Check sheet for the modelled part. Datum: model origin and axes. Units: mm. Face numbers are marked on the shaded views. A direction names the side the tool comes from. Coordinates: 2 decimals unless noted, no trailing zeros. Write each loop counter-clockwise with the first axis right and the second up, starting at its lowest first coordinate (ties: lowest second). Pieces come first, ordered by that corner, then holes. Notation, with made-up numbers: (29.5, -22.75) - (85.5, -22.75) arc R13 ccw to (85.5, -7.75) - close; hole circle Ø3 at (-1, 43). An arc over 180 degrees is marked (long way). Answer as CSV lines item,"result". Start each with the question number.
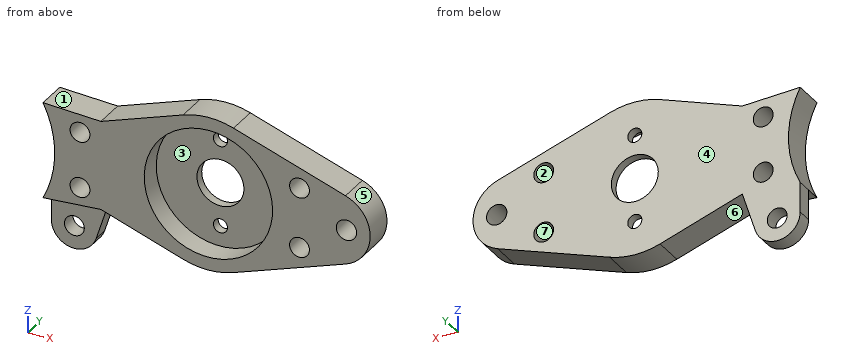
from build123d import *

# Parameters (mm, degrees)
SKETCH1_R           = 1.9
SKETCH1_R_2         = 1.95
BOSS_EXTRUDE1_DEPTH = 6
SKETCH2_R           = 12.3
CUT_EXTRUDE1_DEPTH  = 4.3
SKETCH5_R           = 1.35
SKETCH5_R_2         = 4.5
CUT_EXTRUDE3_DEPTH  = 6
SKETCH6_R           = 1.9
BOSS_EXTRUDE3_DEPTH = 3


with BuildPart() as part:
    # Sketch1 → Boss-Extrude1 (new body)
    with BuildSketch(Plane(origin=(0, 0, 0), x_dir=(1, 0, 0), z_dir=(0, 1, 0))):
        with BuildLine():
            Line((11.089751242, 8.53), (0, 9.208278243))
            ThreePointArc((0, 9.208278243), (2.245912814, 0), (0, -9.208278243))
            Line((0, -9.208278243), (11.089751242, -8.53))
            Line((11.089751242, -8.53), (26.847851363, -13.985564185))
            ThreePointArc((26.847851363, -13.985564185), (31.672879121, -14.799990383), (36.499751242, -13.996567436))
            Line((36.499751242, -13.996567436), (57.964751242, -6.619998112))
            ThreePointArc((57.964751242, -6.619998112), (62.689751242, 0), (57.964751242, 6.619998112))
            Line((57.964751242, 6.619998112), (36.499751242, 13.996567436))
            ThreePointArc((36.499751242, 13.996567436), (31.672879121, 14.799990383), (26.847851363, 13.985564185))
            Line((26.847851363, 13.985564185), (11.089751242, 8.53))
        make_face()
        with Locations(Location((7.089751242, -5.35, 0), (0, 0, 270))):
            Circle(SKETCH1_R, mode=Mode.SUBTRACT)
        with Locations(Location((7.089751242, 5.35, 0), (0, 0, 270))):
            Circle(SKETCH1_R, mode=Mode.SUBTRACT)
        with Locations(Location((49.14768086, 5.75, 0), (0, 0, 270))):
            Circle(SKETCH1_R, mode=Mode.SUBTRACT)
        with Locations(Location((49.14768086, -5.75, 0), (0, 0, 270))):
            Circle(SKETCH1_R, mode=Mode.SUBTRACT)
        with Locations(Location((58.14768086, 0, 0), (0, 0, 270))):
            Circle(SKETCH1_R_2, mode=Mode.SUBTRACT)
    extrude(amount=BOSS_EXTRUDE1_DEPTH)

    # Sketch2 → Cut-Extrude1 (cut)
    with BuildSketch(Plane(origin=(0, 0, 0), x_dir=(1, 0, 0), z_dir=(0, 1, 0))):
        with Locations(Location((31.689751242, 0, 0), (0, 0, 270))):
            Circle(SKETCH2_R)
    extrude(amount=CUT_EXTRUDE1_DEPTH, mode=Mode.SUBTRACT)

    # Sketch5 → Cut-Extrude3 (cut)
    with BuildSketch(Plane(origin=(0, 0, 0), x_dir=(1, 0, 0), z_dir=(0, 1, 0))):
        with Locations(Location((31.689751242, 8.35, 0), (0, 0, 270))):
            Circle(SKETCH5_R)
        with Locations(Location((31.689751242, -8.35, 0), (0, 0, 270))):
            Circle(SKETCH5_R)
        with Locations(Location((31.689751242, 0, 0), (0, 0, 270))):
            Circle(SKETCH5_R_2)
    extrude(amount=CUT_EXTRUDE3_DEPTH, mode=Mode.SUBTRACT)

    # Sketch6 → Boss-Extrude3 (add)
    # profile 1 of 2: a face of its own
    with BuildSketch(Plane(origin=(0, 6, 0), x_dir=(1, 0, 0), z_dir=(0, 1, 0))):
        with BuildLine():
            Line((0, 14.950374836), (0, 9.208278243))
            Line((0, 9.208278243), (11.089751242, 8.53))
            Line((11.089751242, 8.53), (8.588241962, 16.298940471))
            ThreePointArc((8.588241962, 16.298940471), (3.717454995, 19.29711296), (0, 14.950374836))
        make_face()
        with Locations(Location((4.4, 14.950374836, 0), (0, 0, 270))):
            Circle(SKETCH6_R, mode=Mode.SUBTRACT)
    # profile 2 of 2: a face of its own
    with BuildSketch(Plane(origin=(0, 6, 0), x_dir=(1, 0, 0), z_dir=(0, 1, 0))):
        with BuildLine():
            Line((0, 14.950374836), (0, 9.208278243))
            Line((0, 9.208278243), (11.089751242, 8.53))
            Line((11.089751242, 8.53), (8.588241962, 16.298940471))
            ThreePointArc((8.588241962, 16.298940471), (3.717454995, 19.29711296), (0, 14.950374836))
        make_face()
        with Locations(Location((4.4, 14.950374836, 0), (0, 0, 270))):
            Circle(SKETCH6_R, mode=Mode.SUBTRACT)
    extrude(amount=-BOSS_EXTRUDE3_DEPTH)


solid = part.part
(1) Release check for a two-part mould opening along Z. For the marked faces 5, 6 and 7 record: pulls with the +Z half, pulls with the -Z half, needs draft (parallel to the pull), parting line crosses it, or undercut.
(2) Cross-section at B-B on x = 4.4. Record the boundary of the cut face in (y, z).
(3) Tool access check on the marked faces 1, 2, 3 and 4. Record the directions out of +Z, -Z, +X, -X, +Y, -Y that give a thin tool (end or side, any length) a straight path to the whole face; none if there is none.
(4) Material ranges on probe 1 along X at (y, z) = (4.9, 0); probe 2 along Z at (x, y) = (48, 3.7); probe 3 along Z at (x, y) = (50, 2.9), recorded low to high. Write a range as from..to.
(5) Go/stop test with flat-tipped pins: P1, Ø10.5, axis at x = 31.69, z = 0, coming from the -Y side; P2, Ø5, axis at x = 4.4, z = -14.95, coming from the -Y side; P3, Ø19.5, axis at x = 31.69, z = 0, coming from the +Y side. Record where each tip stops, or that it passes through.
(6) Cross-section at A-A on z = 0. Record the boundary of the cut face in (x, y), plus the area to 3 significant figures.
(7) Cross-section at D-D on x = 39. Record the boundary of the cut face in (y, z).
(8) Cross-section at C-C on y = 0.6. Record the boundary of the cut face in (x, z).
Checked values:
1,face 5,"parting line crosses it"
1,face 6,"pulls with the -Z half"
1,face 7,"undercut"
2,outline,"(0, -8.94) - (3, -8.94) - (3, -13.05) - (6, -13.05) - (6, 8.94) - (0, 8.94) - close; (3, -19.35) - (6, -19.35) - (6, -16.85) - (3, -16.85) - close"
3,face 1,"+Z, +Y, -Y"
3,face 2,"+Y, -Y"
3,face 3,"-Y"
3,face 4,"+Z, -Z, +X, -X, +Y"
4,probe 1,"2.25..27.19, 36.19..56.2, 60.1..62.69"
4,probe 2,"-10.04..-7.26, -4.24..4.24, 7.26..10.04"
4,probe 3,"-9.36..-7.45, -4.05..4.05, 7.45..9.36"
5,P1,"y = 4.3"
5,P2,"y = 3"
5,P3,"y = 6"
6,outline,"(2.25, 0) - (19.39, 0) - (19.39, 4.3) - (27.19, 4.3) - (27.19, 6) - (2.25, 6) - close; (36.19, 4.3) - (43.99, 4.3) - (43.99, 0) - (56.2, 0) - (56.2, 6) - (36.19, 6) - close; (60.1, 0) - (62.69, 0) - (62.69, 6) - (60.1, 6) - close"
6,area,"218 mm^2"
7,outline,"(0, -13.14) - (6, -13.14) - (6, 13.14) - (0, 13.14) - (0, 9.89) - (4.3, 9.89) - (4.3, -9.89) - (0, -9.89) - close"
8,outline,"(0, -9.21) - (11.09, -8.53) - (26.85, -13.99) arc R14.8 ccw to (36.5, -14) - (57.96, -6.62) arc R7 ccw to (57.96, 6.62) - (36.5, 14) arc R14.8 ccw to (26.85, 13.99) - (11.09, 8.53) - (0, 9.21) arc R20 cw to start; hole circle Ø3.8 at (7.09, -5.35); hole circle Ø3.8 at (7.09, 5.35); hole circle Ø24.6 at (31.69, 0); hole circle Ø3.8 at (49.15, -5.75); hole circle Ø3.8 at (49.15, 5.75); hole circle Ø3.9 at (58.15, 0)"
